For this review, take the finished solid that the model builds, in its own axes (mm). Face numbers are marked on the shaded views. A direction names the side the tool comes from. Round coordinates to 2 decimals unless told otherwise and drop trailing zeros. Loops run counter-clockwise (first coordinate to the right, second up) from the corner with the lowest first, then second, coordinate; pieces in that order, holes last. Notation, with made-up numbers: (-24, 40) -> (-12, 40) arc R30 ccw to (-12, 76) -> close; hole circle Ø10 at (-11, 25.25). An arc over 180 degrees is marked (long way). One line per question, with ' | ' between items. Start each with the question number.
1. Consider section A-A (x = -25.5). Write out the cut boundary in (y, z).
2. For pin 1 Ø3.5 at (x, z) = (-7, -7.5) entering from +Y; pin 2 Ø0.8 at (x, y) = (3, 21) entering from +Z; pin 3 Ø1.5 at (x, z) = (-25, -9) entering from -Y; pin 4 Ø2 at (x, z) = (-25.5, -9.5) entering from +Y, all flat-tipped, find the tip position at first contact; note any pin that passes through.
3. Consider section C-C (x = -17). Write out the cut boundary in (y, z), and give its area (3 significant figures).
4. Consider section D-D (z = -2.5). Write out the cut boundary in (x, y), and give its area (3 significant figures).
5. Wall thickness on line 1 along Z through (x, y) = (-25.5, 20.35); line 2 along X through (y, z) = (20.95, -2.5); line 3 along Y through (x, z) = (-18.5, -5): over which ranges is each line inside the solid? List them lowest first.
6. Consider section B-B (y = 6). Write out the cut boundary in (x, z), and give its area (3 significant figures).
7. For the marked faces 4, 5 and 6, list the 3-axis set-ups (+Z, -Z, +X, -X, +Y, -Y) from which the entire face can be reached by the end or side of a thin tool; tool diameter is ignored.
8. Draft analysis for pull direction Z (two halves, no side actions). For the marked faces 1, 2 and 3, state which applies: pulls with the +Z half, pulls with the -Z half, needs draft (parallel to the pull), parting line crosses it, or undercut.
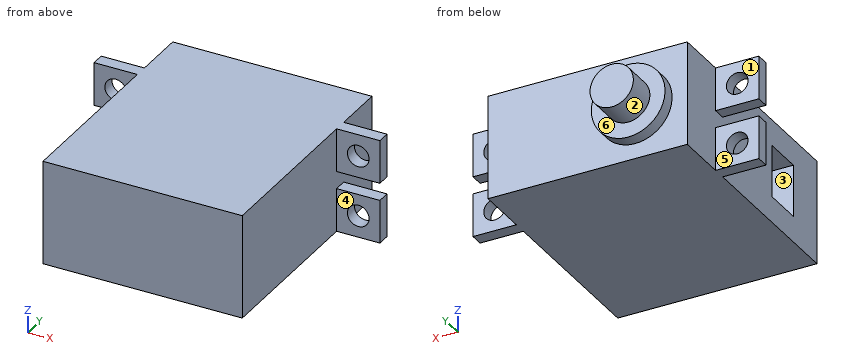
Autodesk Inventor part; units mm, degrees
ref_plane "YZ Plane" through (0, 0, 0) normal (1, 0, 0) x (0, 1, 0)
ref_plane "XZ Plane" through (0, 0, 0) normal (0, 1, 0) x (-1, 0, 0)
ref_plane "XY Plane" through (0, 0, 0) normal (0, 0, 1) x (1, 0, 0)
sketch "Boceto1" plane through (0, 0, 0) normal (0, 1, 0) x (-1, 0, 0)
  line L0 (0, 0) -> (23, 0)
  line L1 (23, 0) -> (23, -12)
  line L2 (23, -12) -> (0, -12)
  line L3 (0, -12) -> (0, 0)
  dimension "d0" = 23
  dimension "d1" = 12
extrude "Extrusión1" add sketch "Boceto1" along normal blind 27.5
sketch "Boceto2" plane through (0, 27.5, 0) normal (0, 1, 0) x (1, 0, 0)
  line L0 (0, 0) -> (0, 12)
  line L1 (0, 0) -> (0, 12)
  line L2 (0, 6) -> (-17, 6)
  circle A0 centre (-17, 6) radius 4.25
  circle A1 centre (-17, 6) radius 2.5
  dimension "d4" = 17
  dimension "d5" = 8.5
  dimension "d6" = 5
extrude "Extrusión2" add sketch "Boceto2" along normal blind 5 contours A1
sketch "Boceto3" plane through (0, 27.5, 0) normal (0, 1, 0) x (1, 0, 0)
  circle A0 centre (-17, 6) radius 2.5
  circle A1 centre (-17, 6) radius 4.25
  point P0 (0, 0)
  dimension "d9" = 8.5
extrude "Extrusión3" add sketch "Boceto3" along normal blind 1.5
sketch "Boceto4" plane through (-23, 0, -12) normal (-1, 0, 0) x (0, 0, 1)
  line L0 (12, 0) -> (12, 27.5)
  line L1 (12, 27.5) -> (12, 20)
  line L2 (12, 20) -> (12, 21.5)
  line L3 (0, 0) -> (0, 27.5)
  line L4 (12, 21.5) -> (7, 21.5)
  line L5 (7, 21.5) -> (7, 20)
  line L6 (7, 20) -> (12, 20)
  line L7 (0, 21.5) -> (5, 21.5)
  line L8 (5, 21.5) -> (5, 20)
  line L9 (5, 20) -> (0, 20)
  line L10 (0, 21.5) -> (0, 20)
  dimension "d12" = 7.5
  dimension "d13" = 1.5
  dimension "d14" = 5
  dimension "d15" = 5
extrude "Extrusión4" add sketch "Boceto4" along normal blind 5 and the other way blind 28
sketch "Boceto5" plane through (-23, 21.5, -7) normal (0, 1, 0) x (1, 0, 0)
  line L0 (-5, 0) -> (-5, 5)
  line L1 (-5, 2.5) -> (0, 2.5)
  line L2 (0, -7) -> (0, 5)
  circle A0 centre (-2.5, 2.5) radius 1.25
  circle A1 centre (-2.5, -4.5) radius 1.25
  line L3 (28, 0) -> (28, 5)
  line L4 (28, 2.5) -> (23, 2.5)
  circle A2 centre (25.5, 2.5) radius 1.25
  circle A3 centre (25.5, -4.5) radius 1.25
  point P0 (23, -7)
  dimension "d20" = 2.5
  dimension "d21" = 2.5
  dimension "d22" = 2.5
  dimension "d23" = 2.5
extrude "Extrusión5" cut sketch "Boceto5" against normal blind 5
sketch "Boceto6" plane through (-23, 0, -12) normal (-1, 0, 0) x (0, 0, 1)
  line L0 (12, 0) -> (12, 20)
  line L1 (12, 20) -> (12, 9.5)
  line L2 (12, 9.5) -> (0, 9.5)
  line L3 (0, 0) -> (0, 20)
  line L4 (6, 9.5) -> (9, 9.5)
  line L5 (9, 9.5) -> (9, 5)
  line L6 (9, 5) -> (3, 5)
  line L7 (3, 5) -> (3, 9.5)
  dimension "d26" = 10.5
  dimension "d27" = 3
  dimension "d28" = 4.5
  dimension "d29" = 6
extrude "Extrusión6" cut sketch "Boceto6" against normal blind 5
properties part number "microservo_FT_2322"
Answer block:
1) outline: (20, -12) -> (21.5, -12) -> (21.5, -10.75) -> (20, -10.75) -> close; (20, -8.25) -> (21.5, -8.25) -> (21.5, -7) -> (20, -7) -> close; (20, -5) -> (21.5, -5) -> (21.5, -3.75) -> (20, -3.75) -> close; (20, -1.25) -> (21.5, -1.25) -> (21.5, 0) -> (20, 0) -> close
2) pin 1: stops at y = 27.5 | pin 2: stops at z = 0 | pin 3: stops at y = 20 | pin 4: passes through
3) outline: (0, -12) -> (27.5, -12) -> (27.5, -10.25) -> (29, -10.25) -> (29, -8.5) -> (32.5, -8.5) -> (32.5, -3.5) -> (29, -3.5) -> (29, -1.75) -> (27.5, -1.75) -> (27.5, 0) -> (0, 0) -> close | area: 360 mm2
4) outline: (-28, 20) -> (-26.75, 20) -> (-26.75, 21.5) -> (-28, 21.5) -> close; (-24.25, 20) -> (-23, 20) -> (-23, 0) -> (0, 0) -> (0, 20) -> (1.25, 20) -> (1.25, 21.5) -> (0, 21.5) -> (0, 27.5) -> (-14.59, 27.5) -> (-14.59, 29) -> (-19.41, 29) -> (-19.41, 27.5) -> (-23, 27.5) -> (-23, 21.5) -> (-24.25, 21.5) -> close; (3.75, 20) -> (5, 20) -> (5, 21.5) -> (3.75, 21.5) -> close | area: 647 mm2
5) line 1: z = -12 to -10.75, -8.25 to -7, -5 to -3.75, -1.25 to 0 | line 2: x = -28 to -26.75, -24.25 to 1.25, 3.75 to 5 | line 3: y = 0 to 5, 9.5 to 32.5
6) outline: (-23, -12) -> (0, -12) -> (0, 0) -> (-23, 0) -> (-23, -3) -> (-18, -3) -> (-18, -9) -> (-23, -9) -> close | area: 246 mm2
7) face 4: +Z, -Z, +X, -Y | face 5: +Z, -Z, -X, +Y | face 6: +Y
8) face 1: needs draft | face 2: parting line crosses it | face 3: undercut
